Autodesk Inventor part; units mm, degrees
ref_plane "Work Plane1" through (-5.6, 5.6, 0) normal (0, 1, 0) x (1, 0, 0)
ref_plane "YZ Plane" through (0, 0, 0) normal (1, 0, 0) x (0, 1, 0)
ref_plane "XZ Plane" through (0, 0, 0) normal (0, 1, 0) x (-1, 0, 0)
sketch "Sketch1" plane through (0, 0, 0) normal (0, 0, 1) x (1, 0, 0)
  circle A0 centre (0, 0) radius 5.6
  dimension "d0" = 11.2
extrude "Extrusion1" add sketch "Sketch1" against normal blind 9
ref_plane "Work Plane1" through (-5.6, 5.6, 0) normal (0, 1, 0) x (1, 0, 0)
sketch "Sketch3" plane through (-5.6, 5.6, 0) normal (0, 1, 0) x (1, 0, 0)
  circle A0 centre (5.6, 4.5) radius 1.2
  point P0 (5.6, 0)
  dimension "d9" = 2.4
hole "Hole1" at (0, 5.6, -4.5) direction (0, -1, 0) diameter 2.459 depth 5.6
sketch "Sketch4" plane through (0, 0, 0) normal (0, 0, 1) x (1, 0, 0)
  circle A0 centre (0, 0) radius 5.6
  circle A1 centre (0, 0) radius 3
  dimension "d17" = 6
extrude "Extrusion3" add sketch "Sketch4" along normal blind 6 contours A1
properties part number "gear motor"
Design review of the part built by this model. Coordinates are the model's own, in mm. A direction names the side the tool comes from. Coordinates: 2 decimals unless noted, no trailing zeros. Order: outer loops, then holes, each group sorted by start corner. A loop starts at its lowest first (then second) coordinate and runs counter-clockwise, first axis right, second up. Notation, with made-up numbers: (12.5, -32.75) -> (20.5, -32.75) arc R8 cw to (20.5, -22.75) -> close; hole circle Ø11 at (62.25, -1). An arc over 180 degrees is marked (long way). One line per item, written item: value.
1) We need section D-D, the plane x = 0.5. Give the boundary of the cut face in (y, z).
Output values:
outline: (-5.58, -9) -> (5.58, -9) -> (5.58, -5.62) -> (0, -5.62) -> (0, -3.38) -> (5.58, -3.38) -> (5.58, 0) -> (2.96, 0) -> (2.96, 6) -> (-2.96, 6) -> (-2.96, 0) -> (-5.58, 0) -> close
2) To check wall thickness, follow probe 1 along Z at (x, y) = (0, 3.25); probe 2 along Z at (x, y) = (0, 1.75); probe 3 along Z at (x, y) = (4.5, -1). State the ranges of each line that lie inside material, in increasing order. Write a range as [from, to].
Output values:
probe 1: z = [-9, -5.73], [-3.27, 0]
probe 2: z = [-9, -5.73], [-3.27, 6]
probe 3: z = [-9, 0]
3) We need section C-C, the plane z = -6.25. Give the boundary of the cut face in (x, y), then the cut area to 3 significant figures.
Output values:
outline: circle Ø11.2 at (0, 0)
area: 98.5 mm2
4) We need section B-B, the plane y = 4. Give the boundary of the cut face in (x, z).
Output values:
outline: (-3.92, -9) -> (3.92, -9) -> (3.92, 0) -> (-3.92, 0) -> close; hole circle Ø2.46 at (0, -4.5)
5) Machinability: for faces 4 (the face through (2.4, -2.4, 0)), 5 (the face through (2.58, -4.97, -4.44)), 6 (the face through (0, 0, -5)), which of the approach directions +Z, -Z, +X, -X, +Y, -Y give a long, thin tool a straight path to every point of the face, cutting with its end or side? Answer none if there is none.
Output values:
face 4: +Z
face 5: +Z, -Z
face 6: +Y
6) We need section A-A, the plane x = 1.75. Give the boundary of the cut face in (y, z), then the cut area to 3 significant figures.
Output values:
outline: (-5.32, -9) -> (5.32, -9) -> (5.32, 0) -> (2.44, 0) -> (2.44, 6) -> (-2.44, 6) -> (-2.44, 0) -> (-5.32, 0) -> close
area: 125 mm2
7) Clearance check with flat-ended pins moving along their axes: P1, Ø2, axis at x = -0.5, z = -4.5, coming from the +Y side; P2, Ø1, axis at y = -4.5, z = 0, coming from the +X side; P3, Ø5, axis at x = -4, z = -6.5, coming from the +Y side. State where each tip first meets the part, or that it passes through.
Output values:
P1: stops at y = 5.55
P2: stops at x = 3.92
P3: stops at y = 5.4
8) Draft analysis for pull direction Z (two halves, no side actions). For faces 1 (the face through (0, 0, 6)), 2 (the face through (0, 0, -9)), 3 (the face through (-0.05, 2.76, -5.73)), state which applies: +Z half, -Z half, draft (parallel to the pull), parting line (faces both ways), or undercut.
Output values:
face 1: +Z half
face 2: -Z half
face 3: undercut
